Check sheet for the modelled part. Datum: model origin and axes. Units: mm. Face numbers are marked on the shaded views. Give positions to 0.01 mm unless a question says otherwise; leave off trailing zeros. Loops run counter-clockwise (first coordinate to the right, second up) from the corner with the lowest first, then second, coordinate; pieces in that order, holes last. Notation, with made-up numbers: (30.25, 55) - (41.25, 55) arc R28 cw to (41.25, 94) - close; hole circle Ø1 at (65.25, 54). An arc over 180 degrees is marked (long way). Use one line per item in the form item = value.
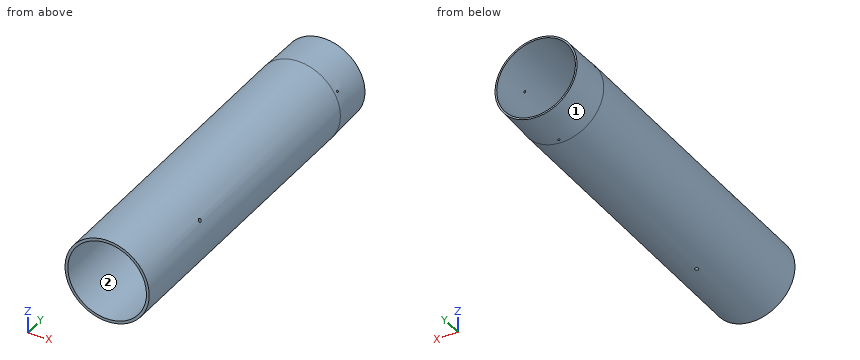
from build123d import *

# Parameters (mm, degrees)
SKETCH1_R                    = 40.8178
SKETCH1_R_2                  = 38.1508
BOSS_EXTRUDE1_DEPTH          = 349.25
SANDING_CHAMFER_SIZE         = 41.275
SANDING_CHAMFER_SIZE2        = 1.044780796
AIRFRAME_BOLT_CUT_REACH      = 364.665
AIRFRAME_BOLT_CUT_END_RADIUS = 38.1508
SKETCH2_R                    = 1.778
AIRFRAME_BOLT_PATTERN_COUNT  = 3
SHEAR_PIN_CUT_REACH          = 364.665
SHEAR_PIN_CUT_END_RADIUS     = 38.1508
SKETCH3_R                    = 0.9906
SHEAR_PIN_PATTERN_COUNT      = 3


with BuildPart() as part:
    # Sketch1 → Boss-Extrude1 (new body)
    with BuildSketch(Plane(origin=(0, 0, 0), x_dir=(1, 0, 0), z_dir=(0, 1, 0))):
        with Locations(Location((0, 0, 0), (0, 0, 270))):
            Circle(SKETCH1_R)
        with Locations(Location((0, 0, 0), (0, 0, 270))):
            Circle(SKETCH1_R_2, mode=Mode.SUBTRACT)
    extrude(amount=BOSS_EXTRUDE1_DEPTH)

    # Sanding Chamfer
    sanding_chamfer_edges = [part.edges().sort_by_distance(p)[0] for p in [
        (0, 349.25, -40.8178),
    ]]
    sanding_chamfer_side = [part.faces().sort_by_distance(p)[0] for p in [
        (0, 174.625, -40.8178),
    ]]
    chamfer(sanding_chamfer_edges, length=SANDING_CHAMFER_SIZE, length2=SANDING_CHAMFER_SIZE2, reference=sanding_chamfer_side[0])

    # Airframe Bolt Cut: up to this cylinder (the profile starts outside it)
    airframe_bolt_cut_end = Plane(origin=(0, 90.4875, 0), z_dir=(0, -1, 0)) * Cylinder(AIRFRAME_BOLT_CUT_END_RADIUS, 806.6316, mode=Mode.PRIVATE)
    # Sketch2 → Airframe Bolt Cut (cut, up to the surface)
    with BuildSketch(Plane(origin=(35.349251727, 0, 20.4089), x_dir=(0, -1, 0), z_dir=(0.866025403784438, 0, 0.500000000000001)), mode=Mode.PRIVATE) as airframe_bolt_cut_sk1:
        with Locations(Location((-90.4875, 0, 0), (0, 0, 90))):
            Circle(SKETCH2_R)
    airframe_bolt_cut_tool1 = extrude(airframe_bolt_cut_sk1.sketch, amount=-AIRFRAME_BOLT_CUT_REACH, mode=Mode.PRIVATE) - airframe_bolt_cut_end
    airframe_bolt_cut = airframe_bolt_cut_tool1.solids().sort_by_distance((35.349252, 90.4875, 20.4089))[0]
    add(airframe_bolt_cut, mode=Mode.SUBTRACT)

    # Airframe Bolt Pattern: Airframe Bolt Cut ×3 about axis
    airframe_bolt_pattern_axis = Axis((0, -55, 0), (0, 1, 0))
    for i in range(1, AIRFRAME_BOLT_PATTERN_COUNT):
        add(airframe_bolt_cut.rotate(airframe_bolt_pattern_axis, i * 360 / AIRFRAME_BOLT_PATTERN_COUNT), mode=Mode.SUBTRACT)

    # Shear Pin Cut: up to this cylinder (the profile starts outside it)
    shear_pin_cut_end = Plane(origin=(0, 312.5216, 0), z_dir=(0, -1, 0)) * Cylinder(SHEAR_PIN_CUT_END_RADIUS, 806.6316, mode=Mode.PRIVATE)
    # Sketch3 → Shear Pin Cut (cut, up to the surface)
    with BuildSketch(Plane(origin=(35.349251727, 0, 20.4089), x_dir=(0, -1, 0), z_dir=(0.866025403784438, 0, 0.500000000000001)), mode=Mode.PRIVATE) as shear_pin_cut_sk1:
        with Locations(Location((-312.5216, 0, 0), (0, 0, 90))):
            Circle(SKETCH3_R)
    shear_pin_cut_tool1 = extrude(shear_pin_cut_sk1.sketch, amount=-SHEAR_PIN_CUT_REACH, mode=Mode.PRIVATE) - shear_pin_cut_end
    shear_pin_cut = shear_pin_cut_tool1.solids().sort_by_distance((35.349252, 312.5216, 20.4089))[0]
    add(shear_pin_cut, mode=Mode.SUBTRACT)

    # Shear Pin Pattern: Shear Pin Cut ×3 about axis
    shear_pin_pattern_axis = Axis((0, -55, 0), (0, 1, 0))
    for i in range(1, SHEAR_PIN_PATTERN_COUNT):
        add(shear_pin_cut.rotate(shear_pin_pattern_axis, i * 360 / SHEAR_PIN_PATTERN_COUNT), mode=Mode.SUBTRACT)


solid = part.part
Item 1: Section check B-B on y = 150.5. Record the boundary of the cut face in (x, z), then the cut area to 3 significant figures.
Answer block:
outline = circle Ø81.64 at (0, 0); hole circle Ø76.3 at (0, 0)
area = 662 mm2
Item 2: Section check A-A on z = 0. Record the boundary of the cut face in (x, y) (3 decimals).
Answer block:
outline = (-40.818, 0) - (-38.151, 0) - (-38.151, 349.25) - (-39.773, 349.25) - (-40.818, 307.975) - close; (38.151, 0) - (40.818, 0) - (40.818, 307.975) - (39.773, 349.25) - (38.151, 349.25) - close
Item 3: Gauge pin test, flat ends, axial feed: P1, Ø2, axis at y = 116, z = -19.5, coming from the -X side; P2, Ø12, axis at x = 16, y = 247, coming from the +Z side; P3, Ø1.5, axis at x = 1, y = 190, coming from the +Z side. Record the tip position at first contact, or that the pin passes through.
Answer block:
P1 = -36.38
P2 = 39.57
P3 = 40.82
Item 4: Thickness scan on L1, parallel to X at y = 119, z = 0; L2, parallel to Z at x = 14, y = 92. Record the ranges inside material, lowest first.
Answer block:
L1 = -40.82 to -38.15, 38.15 to 40.82
L2 = -38.34 to -35.49, 35.49 to 38.34
Item 5: Mould release check, pull along X, two halves, no side actions. Record for the marked faces 1 and 2: released by +X, released by -X, zero draft, split by the parting line, or undercut.
Answer block:
face_1 = split by the parting line
face_2 = undercut
Item 6: Section check C-C on y = 321. Record the boundary of the cut face in (x, z).
Answer block:
outline = circle Ø80.98 at (0, 0); hole circle Ø76.3 at (0, 0)
